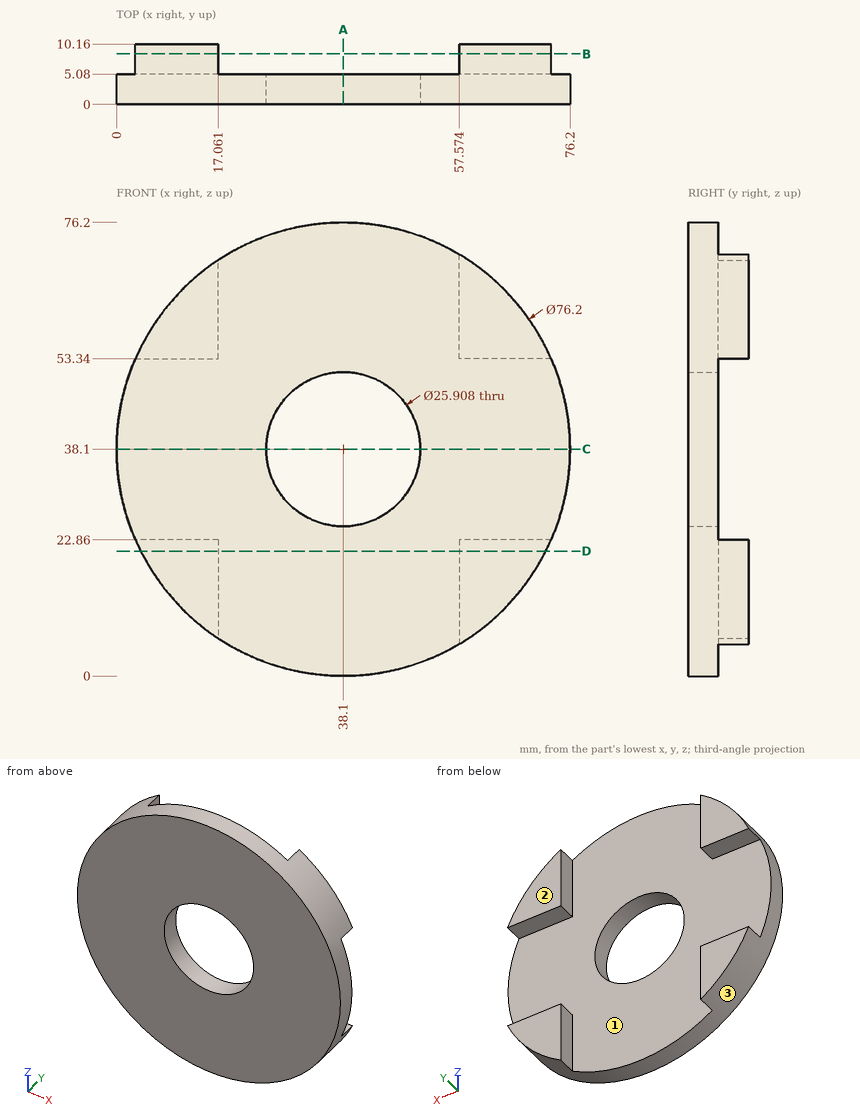
For this review, use the dimensioned drawing (mm, ordinates from the lowest corner) and the shaded views. Round coordinates to 2 decimals unless told otherwise and drop trailing zeros. Write each loop counter-clockwise with the first axis right and the second up, starting at its lowest first coordinate (ties: lowest second). Pieces come first, ordered by that corner, then holes. Notation, with made-up numbers: M 57.5,51 L 110.5,51 A5 ccw 110.5,57 Z; hole C 20.25,-32 d6. An arc over 180 degrees is marked long. Write item = value, one per line. Start each with the question number.
(1) We need section B-B (y = 8.5). Give the boundary of the cut face in (x, z), then the cut area to 3 significant figures.
(2) We need section A-A (x = 38.1). Give the boundary of the cut face in (y, z).
(3) We need section D-D (z = 21). Give the boundary of the cut face in (x, y), then the cut area to 3 significant figures.
(4) Clearance check with flat-ended pins moving along their axes: pin 1 Ø15.5 at (x, z) = (38.1, 38.1) entering from +Y; pin 2 Ø1 at (y, z) = (9, 67.5) entering from +X; pin 3 Ø4 at (x, y) = (66, 7.5) entering from +Z; pin 4 Ø3 at (x, z) = (44.5, 17) entering from +Y. State where each tip first meets the part, or that it passes through.
(5) We need section C-C (z = 38.1). Give the boundary of the cut face in (x, y).
(6) For line 1 along X through (y, z) = (2.4, 38.1); line 2 along Y through (x, z) = (31, 5), list the stretches that pass through material, from the lowest coordinate up.
(7) The part is to be moulded in two halves that separate along X. For the marked faces 1, 2 and 3, say which applies: +X half, -X half, draft (parallel to the pull), parting line (faces both ways), or undercut.
Results found:
q1.outline = M 3.18,22.86 A38.1 ccw 17.06,6.34 L 17.06,22.86 Z; M 3.18,53.34 L 17.06,53.34 L 17.06,69.86 A38.1 ccw Z; M 57.57,5.35 A38.1 ccw 73.02,22.86 L 57.57,22.86 Z; M 57.57,53.34 L 73.02,53.34 A38.1 ccw 57.57,70.85 Z
q1.area = 602 mm²
q2.outline = M 0,0 L 5.08,0 L 5.08,25.15 L 0,25.15 Z; M 0,51.05 L 5.08,51.05 L 5.08,76.2 L 0,76.2 Z
q3.outline = M 4.05,0 L 72.15,0 L 72.15,10.16 L 57.57,10.16 L 57.57,5.08 L 17.06,5.08 L 17.06,10.16 L 4.05,10.16 Z
q3.area = 486 mm²
q4.pin_1 = through
q4.pin_2 = 62.93
q4.pin_3 = 66.04
q4.pin_4 = 5.08
q5.outline = M 0,0 L 25.15,0 L 25.15,5.08 L 0,5.08 Z; M 51.05,0 L 76.2,0 L 76.2,5.08 L 51.05,5.08 Z
q6.line_1 = 0 to 25.15, 51.05 to 76.2
q6.line_2 = 0 to 5.08
q7.face_1 = undercut
q7.face_2 = draft
q7.face_3 = parting line
